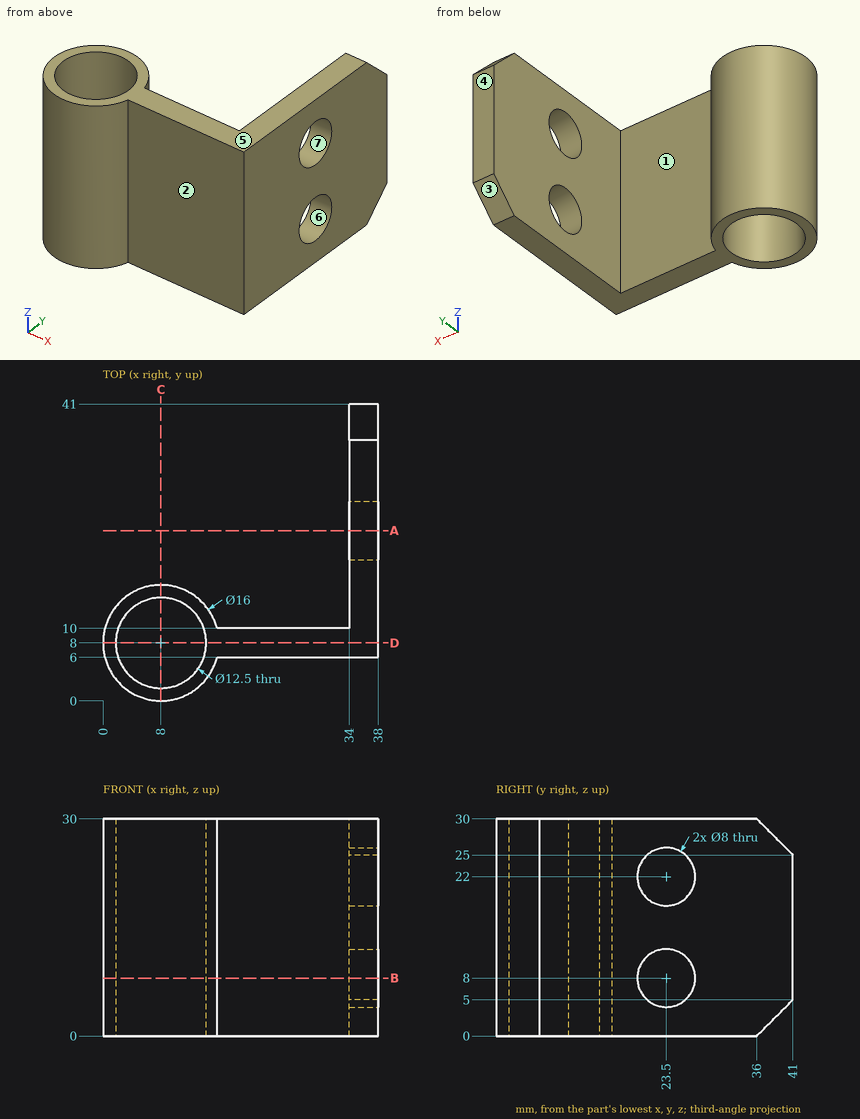
Check sheet for the drawn part. Datum: minimum x, y, z corner. Units: mm. A direction names the side the tool comes from. Coordinates: 2 decimals unless noted, no trailing zeros. Write each loop counter-clockwise with the first axis right and the second up, starting at its lowest first coordinate (ties: lowest second). Pieces come first, ordered by that corner, then holes. Notation, with made-up numbers: M -1.75,45 L 31.25,45 A19 ccw 31.25,49 Z; hole C 35.5,21.5 d3. An arc over 180 degrees is marked long. Use a Markdown table: item, result.
Q1. Sectioned sample at C-C, the plane x = 8. Record the boundary of the cut face in (y, z), plus the area to 3 significant figures.
Reply:
| item | result |
|---|---|
| outline | M 0,0 L 1.75,0 L 1.75,30 L 0,30 Z; M 14.25,0 L 16,0 L 16,30 L 14.25,30 Z |
| area | 105 mm² |
Q2. Sectioned sample at D-D, the plane y = 8. Record the boundary of the cut face in (x, z), plus the area to 3 significant figures.
Reply:
| item | result |
|---|---|
| outline | M 0,0 L 1.75,0 L 1.75,30 L 0,30 Z; M 14.25,0 L 38,0 L 38,30 L 14.25,30 Z |
| area | 765 mm² |
Q3. Draft check along Z on the marked faces 4, 5, 6 and 7. Enter one of: +Z half, -Z half, draft (parallel to the pull), parting line (faces both ways), or undercut.
Reply:
| item | result |
|---|---|
| face 4 | draft |
| face 5 | +Z half |
| face 6 | undercut |
| face 7 | undercut |
Q4. Go/stop test with flat-tipped pins: P1, Ø4, axis at x = 18, z = 15.5, coming from the +Y side; P2, Ø1.5, axis at x = 28.5, z = 22, coming from the -Y side; P3, Ø13, axis at y = 23.5, z = 22, coming from the -X side. Record where each tip stops, or that it passes through.
Reply:
| item | result |
|---|---|
| P1 | stops at y = 10 |
| P2 | stops at y = 6 |
| P3 | stops at x = 34 |
Q5. Sectioned sample at A-A, the plane y = 23.5. Record the boundary of the cut face in (x, z), plus the area to 3 significant figures.
Reply:
| item | result |
|---|---|
| outline | M 34,0 L 38,0 L 38,4 L 34,4 Z; M 34,12 L 38,12 L 38,18 L 34,18 Z; M 34,26 L 38,26 L 38,30 L 34,30 Z |
| area | 56.0 mm² |
Q6. Set-up check for the marked faces 1, 2 and 3: record each of +Z, -Z, +X, -X, +Y, -Y from which the full face is reachable in a straight line by a thin tool's end or side.
Reply:
| item | result |
|---|---|
| face 1 | +Z, -Z, +Y |
| face 2 | +Z, -Z, +X, -Y |
| face 3 | -Z, +X, -X, +Y |
Q7. Sectioned sample at B-B, the plane z = 8. Record the boundary of the cut face in (x, y).
Reply:
| item | result |
|---|---|
| outline | M 15.75,6 L 38,6 L 38,19.5 L 34,19.5 L 34,10 L 15.75,10 A8 ccw long Z; M 34,27.5 L 38,27.5 L 38,41 L 34,41 Z; hole C 8,8 d12.5 |
Q8. Thickness scan on line 1 (Z direction, x = 35.1, y = 23.5); line 2 (Y direction, x = 8, z = 15.5); line 3 (Y direction, x = 26.5, z = 12). Record the ranges inside material, lowest first.
Reply:
| item | result |
|---|---|
| line 1 | z = 0 to 4, 12 to 18, 26 to 30 |
| line 2 | y = 0 to 1.75, 14.25 to 16 |
| line 3 | y = 6 to 10 |
